Verification items for the finished model (mm, model axes). Face numbers are marked on the shaded views. A direction names the side the tool comes from. Give positions to 0.01 mm unless a question says otherwise; leave off trailing zeros. Loops run counter-clockwise (first coordinate to the right, second up) from the corner with the lowest first, then second, coordinate; pieces in that order, holes last. Notation, with made-up numbers: (40.5, 62.5) - (52.5, 62.5) arc R32 ccw to (52.5, 96.5) - close; hole circle Ø7 at (38.5, -25). An arc over 180 degrees is marked (long way). One line per question, with ' | ' between items. Start each with the question number.
1. Section check A-A, the plane z = 0. Enter the section's corners in (x, y), then the cut area to 3 significant figures.
2. Tool access check on the marked faces 4 and 5. Record the directions out of +Z, -Z, +X, -X, +Y, -Y that give a thin tool (end or side, any length) a straight path to the whole face; none if there is none.
3. Mould release check, pull along Z, two halves, no side actions. Record for the marked faces 1, 2 and 3: +Z half, -Z half, draft (parallel to the pull), parting line (faces both ways), or undercut.
4. Section check B-B, the plane y = 9. Enter the section's corners in (x, z).
5. Thickness scan on line 1 along X through (y, z) = (5.75, 0); line 2 along Y through (x, z) = (-17, -7); line 3 along Z through (x, y) = (2, 13). Record the ranges inside material, lowest first. Write a range as from..to.
6. Depth check by flat-ended pin: pin 1 Ø8 at (x, z) = (15, -1.5) entering from +Y; pin 2 Ø3 at (y, z) = (7.5, -11) entering from -X; pin 3 Ø4 at (x, y) = (11.5, 11.5) entering from +Z; pin 4 Ø1.5 at (y, z) = (3, 5) entering from +X. Enter the tip coordinate at first touch or a pass-through.
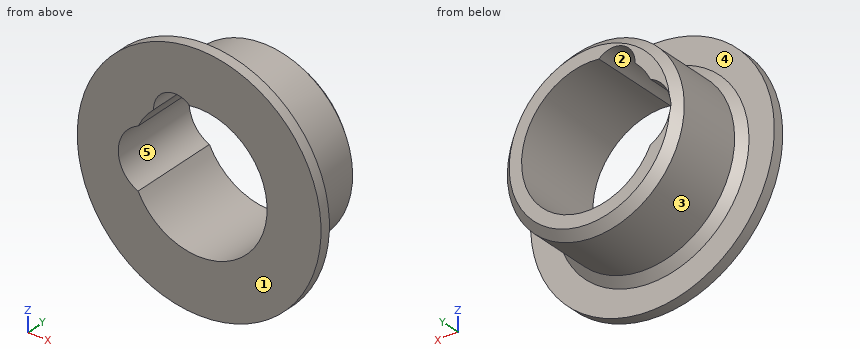
from build123d import *

# Parameters (mm, degrees)
ESBO_O1_R                = 22.6
ESBO_O1_R_2              = 12.6
RESSALTO_EXTRUS_O1_DEPTH = 2
ESBO_O2_R                = 16.4
ESBO_O2_R_2              = 12.6
RESSALTO_EXTRUS_O2_DEPTH = 15
CHANFRO2_SIZE            = 1.5
ESBO_O3_R                = 6
ESBO_O3_R_2              = 4
CORTE_EXTRUS_O1_DEPTH    = 37.201104956


with BuildPart() as part:
    # Esboço1 → Ressalto-extrusão1 (new body)
    with BuildSketch(Plane(origin=(0, 0, 0), x_dir=(1, 0, 0), z_dir=(0, 1, 0))):
        with Locations(Location((0, 0, 0), (0, 0, 270))):
            Circle(ESBO_O1_R)
        with Locations(Location((0, 0, 0), (0, 0, 270))):
            Circle(ESBO_O1_R_2, mode=Mode.SUBTRACT)
    extrude(amount=RESSALTO_EXTRUS_O1_DEPTH)

    # Esboço2 → Ressalto-extrusão2 (add)
    with BuildSketch(Plane(origin=(0, 2, 0), x_dir=(1, 0, 0), z_dir=(0, 1, 0))):
        with Locations(Location((0, 0, 0), (0, 0, 270))):
            Circle(ESBO_O2_R)
        with Locations(Location((0, 0, 0), (0, 0, 270))):
            Circle(ESBO_O2_R_2, mode=Mode.SUBTRACT)
    extrude(amount=RESSALTO_EXTRUS_O2_DEPTH)

    # Chanfro2
    chanfro2_edges = [part.edges().sort_by_distance(p)[0] for p in [
        (0, 17, -16.4),
        (0, 2, -16.4),
    ]]
    chamfer(chanfro2_edges, length=CHANFRO2_SIZE)

    # Esboço3 → Corte-extrusão1 (cut, through all)
    with BuildSketch(Plane(origin=(0, 0, 0), x_dir=(1, 0, 0), z_dir=(0, 1, 0))):
        with Locations((-9, 0)):
            Circle(ESBO_O3_R)
        with Locations((-4.437491748, -9.516231764)):
            Circle(ESBO_O3_R_2)
    extrude(amount=CORTE_EXTRUS_O1_DEPTH, mode=Mode.SUBTRACT)


solid = part.part
Results list:
1) outline: (-22.6, 0) - (-15, 0) - (-15, 16.9) - (-16.4, 15.5) - (-16.4, 3.5) - (-17.9, 2) - (-22.6, 2) - close; (12.6, 0) - (22.6, 0) - (22.6, 2) - (17.9, 2) - (16.4, 3.5) - (16.4, 15.5) - (14.9, 17) - (12.6, 17) - close | area: 113 mm²
2) face 4: +Y | face 5: +Y, -Y
3) face 1: draft | face 2: undercut | face 3: parting line
4) outline: circle Ø32.8 at (0, 0); hole (-11.32, -5.53) arc R12.6 ccw (long way) to (-1.75, 12.48) arc R4 ccw to (-8.43, 9.36) arc R12.6 ccw to (-11.32, 5.53) arc R6 ccw to start
5) line 1: -16.4..-15, 12.6..16.4 | line 2: 0..2 | line 3: -16.28..-12.44, 12.44..16.28
6) pin 1: y = 17 | pin 2: x = -13.37 | pin 3: z = 13.37 | pin 4: x = 16.96
